Part model, mm, in its own coordinate system. Face numbers are marked on the shaded views. A direction names the side the tool comes from. Coordinates: 2 decimals unless noted, no trailing zeros. Loops run counter-clockwise (first coordinate to the right, second up) from the corner with the lowest first, then second, coordinate; pieces in that order, holes last. Notation, with made-up numbers: M 65,-15.5 L 123,-15.5 A12 cw 123,-3.5 Z; hole C -13,-35 d10. An arc over 180 degrees is marked long. Answer as a JSON object with one key per item and string values. Group by question number.
1. Saw through at A-A on z = 0. Write the cut outline in (x, y).
2. Drill centre lines: L1, parallel to Z at x = 0, y = 33; L2, parallel to Y at x = -1.5, z = -1.25; L3, parallel to X at y = 89.5, z = 1.5. Where is each one in solid material? Low to high.
3. Saw through at C-C on y = 27.5. Write the cut outline in (x, z).
4. Mould opens along Z. For the marked faces 3 and 4 say: released by +Z, released by -Z, zero draft, split by the parting line, or undercut.
5. Saw through at D-D on y = -94. Write the cut outline in (x, z).
6. Drop flat-ended pins along their axis: pin 1 Ø5 at (y, z) = (-86, 6.5) entering from -X; pin 2 Ø1.5 at (x, y) = (3, -66.5) entering from -Z; pin 3 Ø10 at (x, y) = (5, 8.5) entering from -Z. Give the stop position or say it passes through.
7. 3-axis set-ups, long thin cutter, end or side, ignore diameter. For the marked faces 1 and 2: which of +Z, -Z, +X, -X, +Y, -Y reach the whole face in a straight line?
8. Saw through at B-B on x = 0. Write the cut outline in (y, z), then the cut area to 3 significant figures.
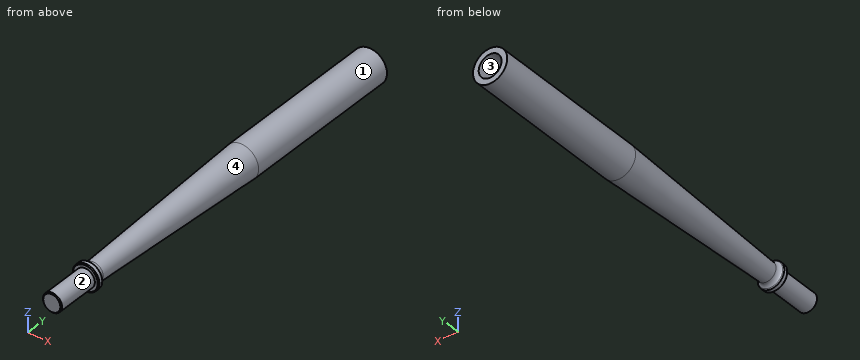
from build123d import *

# Parameters (mm, degrees)
F2_R     = 6
F3_DEPTH = 100
F4_SIZE  = 0.5


# Not quite as in the source:
# - a fillet or chamfer that OpenCascade refuses, or shapes differently, is made with other operations: its cross-section is extruded or revolved along the edge and cut away or added


with BuildPart() as f1:
    # F0 (on Right) → F1 (revolve)
    with BuildSketch(Plane.YZ):
        Polygon((108.9967988729, 0), (108.9967988729, 9), (20.9967988729, 9), (-83.0032011271, 5), (-83.0032011271, 7), (-86.0032011271, 7), (-86.0032011271, 5), (-109.0032011271, 5), (-109.0032011271, 0), align=None)
    revolve(axis=Axis((0, -0.0032011271, 0), (0, -1, 0)))

    # F2 (on face) → F3 (cut)
    with BuildSketch(Plane(origin=(0, 108.9967988729, 0), x_dir=(-1, 0, 0), z_dir=(0, 1, 0))):
        Circle(F2_R)
    extrude(amount=-F3_DEPTH, mode=Mode.SUBTRACT)

    # F4
    f4_edges = [f1.edges().sort_by_distance(p)[0] for p in [
        (0, -109.003201, -5),
        (0, -83.003201, -7),
        (0, -86.003201, -7),
    ]]
    chamfer(f4_edges, length=F4_SIZE)

    # F5: fillet of radius 3 on 1 edges, made by hand

    # F5_s1 → F5_t2 (revolve)
    with BuildSketch(Plane.YZ):
        with BuildLine():
            ThreePointArc((-83.0032011271, 6.5), (-81.8638498753, 5.4457220241), (-80.350077034, 5.1020432343))
            Line((-80.350077034, 5.1020432343), (-80.3477710467, 5.0420875639))
            Line((-80.3477710467, 5.0420875639), (-83.0008951397, 4.9400443295))
            Line((-83.0008951397, 4.9400443295), (-83.0632011271, 5))
            ThreePointArc((-83.0632011271, 5), (-83.0632011271, 5.75), (-83.0539576216, 6.4680034648))
            Line((-83.0539576216, 6.4680034648), (-83.0032011271, 6.5))
        make_face()
    revolve(axis=Axis((0, -83.0032011271, 0), (0, -1, 0)))


solid = f1.part
Outcome:
{
 "1": {"outline": "M -9,21 L -5.1,-80.35 A3 cw -6.5,-83 L -7,-83.5 L -7,-85.5 L -6.5,-86 L -5,-86 L -5,-108.5 L -4.5,-109 L 4.5,-109 L 5,-108.5 L 5,-86 L 6.5,-86 L 7,-85.5 L 7,-83.5 L 6.5,-83 A3 cw 5.1,-80.35 L 9,21 L 9,109 L 6,109 L 6,9 L -6,9 L -6,109 L -9,109 Z"},
 "2": {"L1": "z = -9 to -6, 6 to 9", "L2": "y = -109 to 9", "L3": "x = -8.87 to -5.81, 5.81 to 8.87"},
 "3": {"outline": "C 0,0 d18; hole C 0,0 d12"},
 "4": {"face 3": "undercut", "face 4": "split by the parting line"},
 "5": {"outline": "C 0,0 d10"},
 "6": {"pin 1": "stops at x = -5.71", "pin 2": "stops at z = -5.17", "pin 3": "stops at z = -8.59"},
 "7": {"face 1": "+Y, -Y", "face 2": "-Y"},
 "8": {"outline": "M -109,-4.5 L -108.5,-5 L -86,-5 L -86,-6.5 L -85.5,-7 L -83.5,-7 L -83,-6.5 A3 cw -80.35,-5.1 L 21,-9 L 109,-9 L 109,-6 L 9,-6 L 9,6 L 109,6 L 109,9 L 21,9 L -80.35,5.1 A3 cw -83,6.5 L -83.5,7 L -85.5,7 L -86,6.5 L -86,5 L -108.5,5 L -109,4.5 Z", "area": "2,110 mm²"}
}
